Part print with two shaded views. Sizes in mm from the minimum x, y, z corner. A direction names the side the tool comes from. Coordinates: 2 decimals unless noted, no trailing zeros. Write each loop counter-clockwise with the first axis right and the second up, starting at its lowest first coordinate (ties: lowest second). Pieces come first, ordered by that corner, then holes. Notation, with made-up numbers: (-34.5, 28) - (-30.5, 28) arc R25 ccw to (-30.5, 52) - close; hole circle Ø8 at (-32, 79). An arc over 180 degrees is marked (long way). Answer in a Markdown table with one row per item. Add a question column.
Q1. Band-saw the part on A-A (y = 3.75). List the corners of the cut face in (x, z), and give its area (3 significant figures).
Q2. Two-plate mould, pull along Z, no slides. Class the marked faces 3, 4, 5 and 6: +Z half, -Z half, draft (parallel to the pull), parting line (faces both ways), or undercut.
Q3. Pin check, flat tips, straight feed: pin 1 (1.5 mm diameter, centred on y = 3.5, z = 1.5, fed in from +X); pin 2 (1 mm diameter, centred on x = 5, z = 1, fed in from -Y). Stop position of each tip, or through.
Q4. 3-axis set-ups, long thin cutter, end or side, ignore diameter. For the marked faces 1 and 2: which of +Z, -Z, +X, -X, +Y, -Y reach the whole face in a straight line?
Q5. Drill centre lines: line 1 along Z through (x, y) = (3.25, 5.25); line 2 along X through (y, z) = (5.5, 5); line 3 along X through (y, z) = (1.75, 2.25). Where is each one in solid material? Low to high. Write a range as from..to.
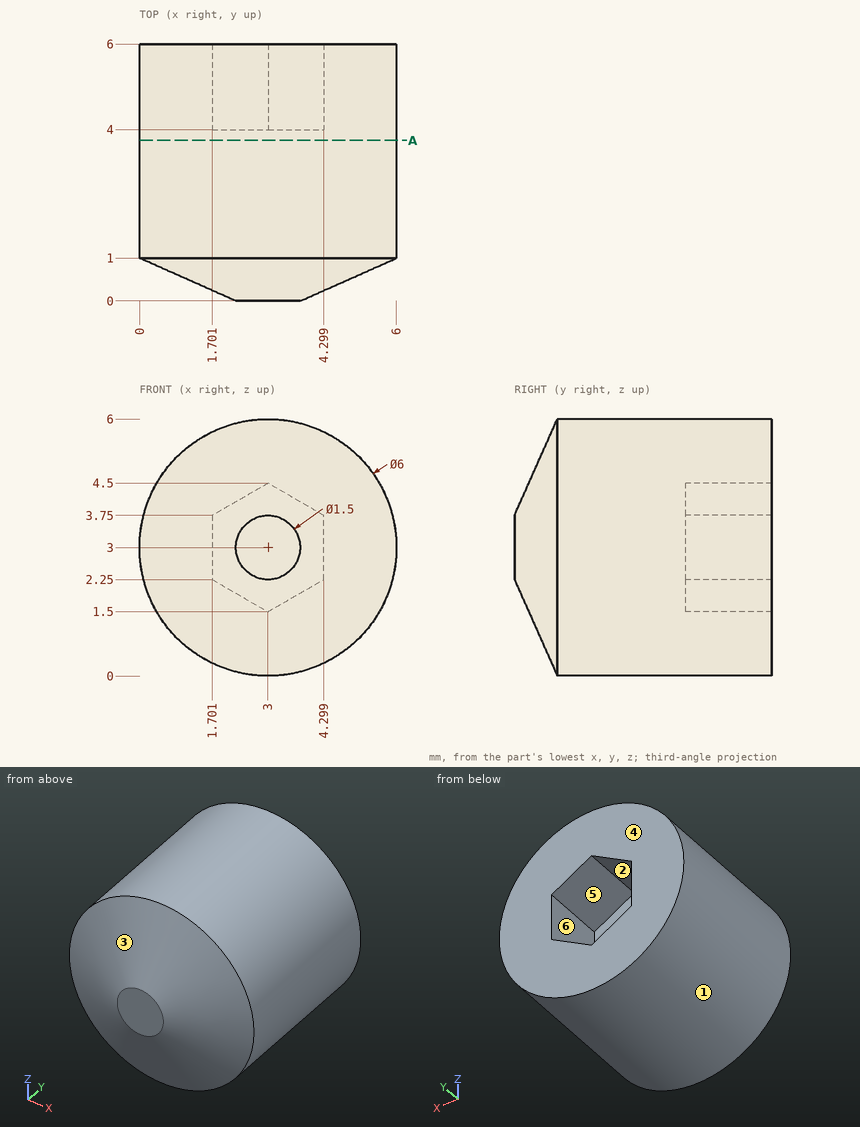
Checked values:
| question | item | result |
|---|---|---|
| 1 | outline | circle Ø6 at (3, 3) |
| 1 | area | 28.3 mm² |
| 2 | face 3 | parting line |
| 2 | face 4 | draft |
| 2 | face 5 | undercut |
| 2 | face 6 | undercut |
| 3 | pin 1 | stops at x = 5.9 |
| 3 | pin 2 | stops at y = 0.7 |
| 4 | face 1 | +Y, -Y |
| 4 | face 2 | +Y |
| 5 | line 1 | z = 0.01..1.64, 4.36..5.99 |
| 5 | line 2 | x = 0.76..5.24 |
| 5 | line 3 | x = 0.1..5.9 |
